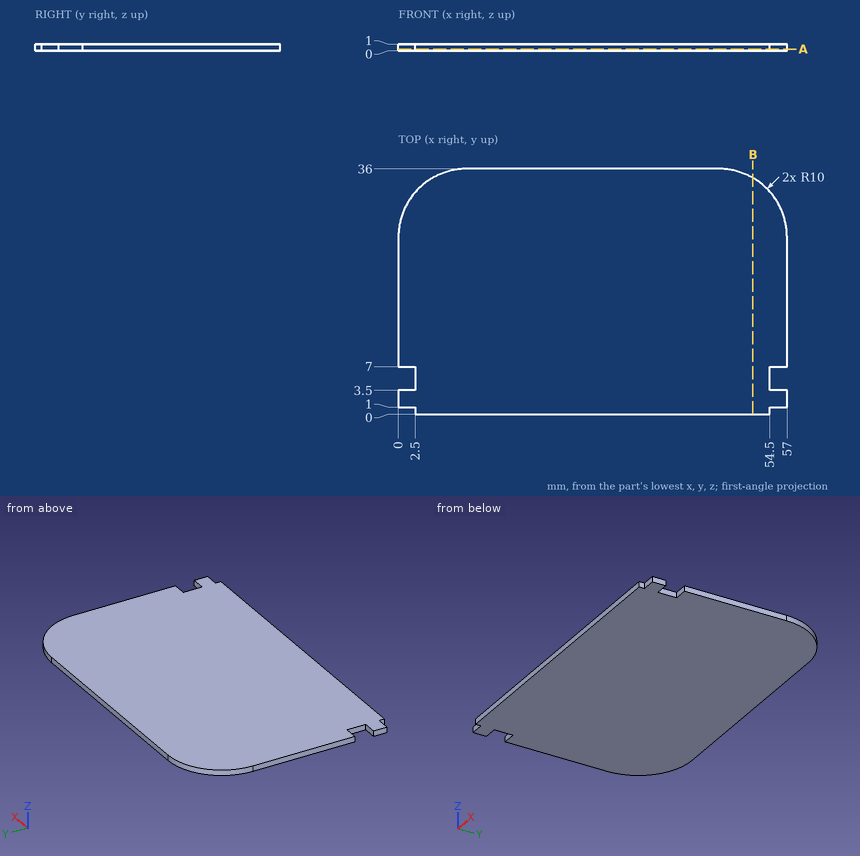
Print and shaded views of the part. All mm, measured from the part's lowest x, y and z. Round coordinates to 2 decimals unless told otherwise and drop trailing zeros. Write each loop counter-clockwise with the first axis right and the second up, starting at its lowest first coordinate (ties: lowest second). Pieces come first, ordered by that corner, then holes. Notation, with made-up numbers: (11.25, -3.5) -> (52.25, -3.5) arc R30 ccw to (52.25, 24.5) -> close; hole circle Ø10 at (21, -36). An arc over 180 degrees is marked (long way). Answer in a Markdown table with one row per item. Add a question column.
Item 1: Drill centre lines: line 1 (X direction, y = 4, z = 0.65); line 2 (Y direction, x = 6.5, z = 0.85); line 3 (X direction, y = 28, z = 0.1). Where is each one in solid material? Low to high. Write a range as from..to.
Item 2: Saw through at B-B, the plane x = 52. Write the cut outline in (y, z).
Item 3: Saw through at A-A, the plane z = 0.25. Write the cut outline in (x, y), then the cut area to 3 significant figures.
Findings below:
| question | item | result |
|---|---|---|
| 1 | line 1 | x = 2.5..54.5 |
| 1 | line 2 | y = 0..35.37 |
| 1 | line 3 | x = 0.2..56.8 |
| 2 | outline | (0, 0) -> (34.66, 0) -> (34.66, 1) -> (0, 1) -> close |
| 3 | outline | (0, 1) -> (2.5, 1) -> (2.5, 0) -> (54.5, 0) -> (54.5, 1) -> (57, 1) -> (57, 3.5) -> (54.5, 3.5) -> (54.5, 7) -> (57, 7) -> (57, 26) arc R10 ccw to (47, 36) -> (10, 36) arc R10 ccw to (0, 26) -> (0, 7) -> (2.5, 7) -> (2.5, 3.5) -> (0, 3.5) -> close |
| 3 | area | 1,990 mm^2 |
